Geometry check sheet. Reference: the model listing, model coordinates, mm. Face numbers are marked on the shaded views. A direction names the side the tool comes from. Give positions to 0.01 mm unless a question says otherwise; leave off trailing zeros. Loops run counter-clockwise (first coordinate to the right, second up) from the corner with the lowest first, then second, coordinate; pieces in that order, holes last. Notation, with made-up numbers: (-35.75, -7.5) -> (-25.75, -7.5) arc R20 cw to (-25.75, 17.5) -> close; hole circle Ø6 at (-5.75, 18.5). An arc over 180 degrees is marked (long way). Write each question's results on one line, items separated by ' | '. Start each with the question number.
1) Scan lines: line 1 (X direction, y = -6.65, z = -18.37); line 2 (Y direction, x = 3, z = 0); line 3 (Z direction, x = -2.05, y = -8.1). Record each from-to range of solid material in increasing order. Write a range as from..to.
2) Sectioned sample at C-C on x = -11.05. Record the cut outline in (y, z).
3) Depth check by flat-ended pin: pin 1 (2 mm diameter, centred on x = -15, y = -7.5, fed in from -Z); pin 2 (12 mm diameter, centred on x = -14.5, z = -30.5, fed in from -Y); pin 3 (1.1 mm diameter, centred on x = 1.5, y = -12, fed in from +Z). Enter the tip coordinate at first touch or a pass-through.
4) Sectioned sample at B-B on x = 7. Record the cut outline in (y, z), then the cut area to 3 significant figures.
5) Draft check along Y on the marked faces 1, 2 and 3. Enter one of: pulls with the +Y half, pulls with the -Y half, needs draft (parallel to the pull), parting line crosses it, or undercut.
6) Set-up check for the marked faces 4 and 5: record each of +Z, -Z, +X, -X, +Y, -Y from which the full face is reachable in a straight line by a thin tool's end or side.
7) Sectioned sample at A-A on x = 12.55. Record the cut outline in (y, z).
8) Sectioned sample at D-D on z = -47. Record the cut outline in (x, y).
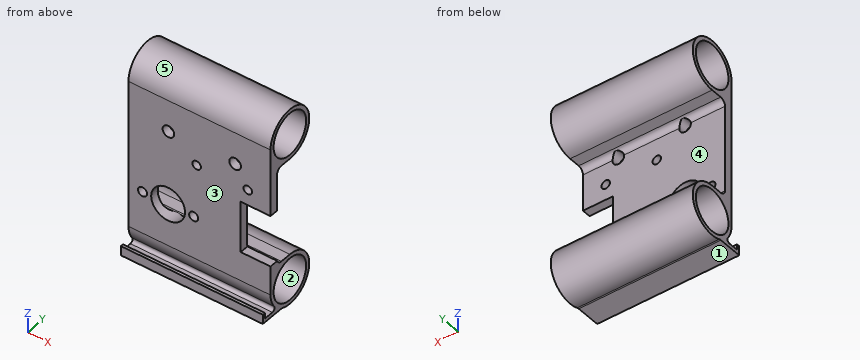
```python
from build123d import *

# Parameters (mm, degrees)
EXTRUDE_1_DEPTH      = 25
EXTRUDE_1_DEPTH_BACK = 25
SKETCH_1_R           = 7.5
SKETCH_2_R           = 1.6
SKETCH_2_R_2         = 5.95
SKETCH_2_W           = 10.49
SKETCH_2_H           = 18.16
EXTRUDE_2_DEPTH      = 25
SKETCH_3_R           = 2.05
EXTRUDE_3_DEPTH      = 25
SKETCH_4_R           = 1.5
EXTRUDE_4_DEPTH      = 10


with BuildPart() as part:
    # Эскиз1 → Выдавливание1 (new, two sides: drawn at the far end of the back side and taken through both)
    with BuildSketch(Plane.YZ.offset(-EXTRUDE_1_DEPTH_BACK)):
        with BuildLine():
            Line((-8.91, -52.3), (-8.91, 0))
            ThreePointArc((-8.91, 0), (6.30032142, 6.30032142), (0, -8.91))
            Line((0, -8.91), (-3.91, -8.91))
            ThreePointArc((-3.91, -8.91), (-5.324213562, -9.495786438), (-5.91, -10.91))
            Line((-5.91, -10.91), (-5.91, -41.39))
            ThreePointArc((-5.91, -41.39), (-5.324213562, -42.804213562), (-3.91, -43.39))
            Line((-3.91, -43.39), (0, -43.39))
            ThreePointArc((0, -43.39), (8.753455219, -53.962865516), (-3.2672994, -60.589321723))
            ThreePointArc((-3.2672994, -60.589321723), (-3.627441686, -60.48513912), (-4.000699939, -60.45))
            Line((-4.000699939, -60.45), (-12.45, -60.45))
            Line((-12.45, -60.45), (-12.45, -57.11))
            Line((-12.45, -57.11), (-11.45, -57.11))
            Line((-11.45, -57.11), (-11.45, -59.11))
            Line((-11.45, -59.11), (-8.028200296, -59.11))
            ThreePointArc((-8.028200296, -59.11), (-7.137617204, -58.564820575), (-7.218089268, -57.523723512))
            ThreePointArc((-7.218089268, -57.523723512), (-8.476475546, -55.045443919), (-8.91, -52.3))
        make_face()
        with Locations(Location((0, 0, 0), (0, 0, 270))):
            Circle(SKETCH_1_R, mode=Mode.SUBTRACT)
        with Locations(Location((0, -52.3, 0), (0, 0, 270))):
            Circle(SKETCH_1_R, mode=Mode.SUBTRACT)
    extrude(amount=EXTRUDE_1_DEPTH + EXTRUDE_1_DEPTH_BACK)

    # Эскиз2 → Выдавливание2 (cut, symmetric)
    with BuildSketch(Plane(origin=(-25, -5.91, -8.91), x_dir=(1, 0, 0), z_dir=(0, 1, 0))):
        with Locations(Location((4.95, 28.46, 0), (0, 0, 90))):
            Circle(SKETCH_2_R)
        with Locations(Location((22.95, 28.46, 0), (0, 0, 90))):
            Circle(SKETCH_2_R)
        with Locations(Location((13.95, 28.46, 0), (0, 0, 137.496887959))):
            Circle(SKETCH_2_R_2)
        with Locations((44.755, 24.01)):
            Rectangle(SKETCH_2_W, SKETCH_2_H)
    extrude(amount=EXTRUDE_2_DEPTH, both=True, mode=Mode.SUBTRACT)

    # Эскиз3 → Выдавливание3 (cut, symmetric)
    with BuildSketch(Plane(origin=(0, -5.91, 0), x_dir=(-1, 0, 0), z_dir=(0, 1, 0))):
        with Locations(Location((10.95, -11.14, 0), (0, 0, 6.441870255))):
            Circle(SKETCH_3_R)
        with Locations(Location((-12.55, -11.14, 0), (0, 0, 6.441870255))):
            Circle(SKETCH_3_R)
    extrude(amount=EXTRUDE_3_DEPTH, both=True, mode=Mode.SUBTRACT)

    # Эскиз4 → Выдавливание4 (cut)
    with BuildSketch(Plane(origin=(0, -5.91, 0), x_dir=(-1, 0, 0), z_dir=(0, 1, 0))):
        with Locations(Location((-17, -18.37, 0), (0, 0, 90))):
            Circle(SKETCH_4_R)
        with Locations(Location((1, -18.37, 0), (0, 0, 90))):
            Circle(SKETCH_4_R)
    extrude(amount=-EXTRUDE_4_DEPTH, mode=Mode.SUBTRACT)


solid = part.part
```
Result:
1) line 1: -25..-2.5, 0.5..15.5, 18.5..25 | line 2: -8.91..-7.5, 7.5..8.91 | line 3: -60.45..-59.11, -56.01..-38.97, -35.77..-19.44, -17.3..3.71
2) outline: (-12.45, -60.45) -> (-4, -60.45) arc R2 cw to (-3.27, -60.59) arc R8.91 ccw (long way) to (0, -43.39) -> (-3.91, -43.39) arc R2 cw to (-4.43, -43.32) -> (-8.91, -43.32) -> (-8.91, -52.3) arc R8.91 ccw to (-7.22, -57.52) arc R1 cw to (-8.03, -59.11) -> (-11.45, -59.11) -> (-11.45, -57.11) -> (-12.45, -57.11) -> close; (-8.91, -31.42) -> (-5.91, -31.42) -> (-5.91, -13.19) -> (-8.91, -13.19) -> close; (-8.91, -9.09) -> (-4.74, -9.09) arc R2 cw to (-3.91, -8.91) -> (0, -8.91) arc R8.91 ccw (long way) to (-8.91, 0) -> close; hole circle Ø15 at (0, -52.3); hole circle Ø15 at (0, 0)
3) pin 1: z = -60.45 | pin 2: y = -8.91 | pin 3: z = -57.11
4) outline: (-12.45, -60.45) -> (-4, -60.45) arc R2 cw to (-3.27, -60.59) arc R8.91 ccw (long way) to (0, -43.39) -> (-3.91, -43.39) arc R2 cw to (-5.91, -41.39) -> (-5.91, -10.91) arc R2 cw to (-3.91, -8.91) -> (0, -8.91) arc R8.91 ccw (long way) to (-8.91, 0) -> (-8.91, -52.3) arc R8.91 ccw to (-7.22, -57.52) arc R1 cw to (-8.03, -59.11) -> (-11.45, -59.11) -> (-11.45, -57.11) -> (-12.45, -57.11) -> close; hole circle Ø15 at (0, -52.3); hole circle Ø15 at (0, 0) | area: 298 mm^2
5) face 1: needs draft | face 2: undercut | face 3: pulls with the -Y half
6) face 4: +X, -X, +Y | face 5: +X, -X
7) outline: (-12.45, -60.45) -> (-4, -60.45) arc R2 cw to (-3.27, -60.59) arc R8.91 ccw (long way) to (0, -43.39) -> (-3.91, -43.39) arc R2 cw to (-5.91, -41.39) -> (-5.91, -13.19) -> (-8.91, -13.19) -> (-8.91, -52.3) arc R8.91 ccw to (-7.22, -57.52) arc R1 cw to (-8.03, -59.11) -> (-11.45, -59.11) -> (-11.45, -57.11) -> (-12.45, -57.11) -> close; (-8.91, -9.09) -> (-4.74, -9.09) arc R2 cw to (-3.91, -8.91) -> (0, -8.91) arc R8.91 ccw (long way) to (-8.91, 0) -> close; hole circle Ø15 at (0, -52.3); hole circle Ø15 at (0, 0)
8) outline: (-25, -8.91) -> (25, -8.91) -> (25, -5.31) -> (-25, -5.31) -> close; (-25, 5.31) -> (25, 5.31) -> (25, 7.16) -> (-25, 7.16) -> close
